from build123d import *

# Parameters (mm, degrees)
F0_W     = 3
F0_H     = 0.7113954189
F0_H_2   = 11.7951147258
F1_DEPTH = 2
F2_R     = 2
F3_W     = 4
F3_H     = 7.7592988014
F3_R     = 0.75
F4_DEPTH = 3
F5_R     = 1.99999


# Not quite as in the source:
# - a fillet or chamfer is up to 0.001 mm smaller than in the source, because OpenCascade refuses the exact size


with BuildPart() as f1:
    # F0 (on Top) → F1 (new body)
    with BuildSketch(Plane.XY):
        with BuildLine():
            ThreePointArc((-21.4, 5.9), (-20.3393398282, 6.3393398282), (-19.9, 7.4))
            Line((-19.9, 7.4), (-20.8, 7.4))
            ThreePointArc((-20.8, 7.4), (-20.9757359313, 6.9757359313), (-21.4, 6.8))
            Line((-21.4, 6.8), (-21.4, 5.9))
        make_face()
        with BuildLine():
            Line((-20.8, 7.4), (-19.9, 7.4))
            ThreePointArc((-19.9, 7.4), (-22.4606601718, 8.4606601718), (-21.4, 5.9))
            Line((-21.4, 5.9), (-21.4, 6.8))
            ThreePointArc((-21.4, 6.8), (-21.8242640687, 7.8242640687), (-20.8, 7.4))
        make_face()
        with BuildLine():
            Line((19.9, 7.4), (-19.9, 7.4))
            ThreePointArc((-19.9, 7.4), (-20.3393398282, 6.3393398282), (-21.4, 5.9))
            Line((-21.4, 5.9), (-21.4, -5.9))
            ThreePointArc((-21.4, -5.9), (-20.3393398282, -6.3393398282), (-19.9, -7.4))
            Line((-19.9, -7.4), (19.9, -7.4))
            ThreePointArc((19.9, -7.4), (20.0395252165, -6.7682497618), (20.4321444846, -6.2540263086))
            Line((20.4321444846, -6.2540263086), (20.4321444846, 6.2540263086))
            ThreePointArc((20.4321444846, 6.2540263086), (20.0395252165, 6.7682497618), (19.9, 7.4))
        make_face()
        Polygon((-1.5, 5.8975573629), (-1.5, 6.6089527819), (1.5, 6.6089527819), (1.5, 5.8975573629), (20.1555918902, 5.8975573629), (20.1555918902, -5.8975573629), (1.5, -5.8975573629), (1.5, -6.6089527819), (-1.5, -6.6089527819), (-1.5, -5.8975573629), (-20.1555918902, -5.8975573629), (-20.1555918902, 5.8975573629), align=None, mode=Mode.SUBTRACT)
        with BuildLine():
            ThreePointArc((22.9, 7.4), (21.4, 8.9), (19.9, 7.4))
            Line((19.9, 7.4), (20.8, 7.4))
            ThreePointArc((20.8, 7.4), (21.4, 8), (22, 7.4))
            ThreePointArc((22, 7.4), (21.8242640687, 6.9757359313), (21.4, 6.8))
            Line((21.4, 6.8), (21.4, 5.9))
            ThreePointArc((21.4, 5.9), (22.4606601718, 6.3393398282), (22.9, 7.4))
        make_face()
        with BuildLine():
            Line((20.8, 7.4), (19.9, 7.4))
            ThreePointArc((19.9, 7.4), (20.0395252165, 6.7682497618), (20.4321444846, 6.2540263086))
            ThreePointArc((20.4321444846, 6.2540263086), (20.8847139324, 5.9912841775), (21.4, 5.9))
            Line((21.4, 5.9), (21.4, 6.8))
            ThreePointArc((21.4, 6.8), (20.9757359313, 6.9757359313), (20.8, 7.4))
        make_face()
        with BuildLine():
            ThreePointArc((21.4, 5.9), (20.8847139324, 5.9912841775), (20.4321444846, 6.2540263086))
            Line((20.4321444846, 6.2540263086), (20.4321444846, -6.2540263086))
            ThreePointArc((20.4321444846, -6.2540263086), (20.8847139324, -5.9912841775), (21.4, -5.9))
            Line((21.4, -5.9), (21.4, 5.9))
        make_face()
        with BuildLine():
            ThreePointArc((-19.9, -7.4), (-20.3393398282, -6.3393398282), (-21.4, -5.9))
            Line((-21.4, -5.9), (-21.4, -6.8))
            ThreePointArc((-21.4, -6.8), (-20.9757359313, -6.9757359313), (-20.8, -7.4))
            Line((-20.8, -7.4), (-19.9, -7.4))
        make_face()
        with BuildLine():
            Line((-21.4, -6.8), (-21.4, -5.9))
            ThreePointArc((-21.4, -5.9), (-22.4606601718, -8.4606601718), (-19.9, -7.4))
            Line((-19.9, -7.4), (-20.8, -7.4))
            ThreePointArc((-20.8, -7.4), (-21.8242640687, -7.8242640687), (-21.4, -6.8))
        make_face()
        with BuildLine():
            ThreePointArc((21.4, -5.9), (20.8847139324, -5.9912841775), (20.4321444846, -6.2540263086))
            ThreePointArc((20.4321444846, -6.2540263086), (20.0395252165, -6.7682497618), (19.9, -7.4))
            Line((19.9, -7.4), (20.8, -7.4))
            ThreePointArc((20.8, -7.4), (20.9757359313, -6.9757359313), (21.4, -6.8))
            Line((21.4, -6.8), (21.4, -5.9))
        make_face()
        with BuildLine():
            ThreePointArc((22.9, -7.4), (22.4606601718, -6.3393398282), (21.4, -5.9))
            Line((21.4, -5.9), (21.4, -6.8))
            ThreePointArc((21.4, -6.8), (21.8242640687, -6.9757359313), (22, -7.4))
            ThreePointArc((22, -7.4), (21.4, -8), (20.8, -7.4))
            Line((20.8, -7.4), (19.9, -7.4))
            ThreePointArc((19.9, -7.4), (21.4, -8.9), (22.9, -7.4))
        make_face()
        with Locations((0, 6.2532550724)):
            Rectangle(F0_W, F0_H)
        with Locations((0, -6.2532550724)):
            Rectangle(F0_W, F0_H)
        Rectangle(F0_W, F0_H_2)
    extrude(amount=F1_DEPTH)

    # F2
    f2_edges = [f1.edges().sort_by_distance(p)[0] for p in [
        (-19.9, 7.4, 1),
        (-19.9, -7.4, 1),
        (-1.5, -5.897557, 1),
        (-20.155592, -5.897557, 1),
        (-20.155592, 5.897557, 1),
        (20.155592, 5.897557, 1),
        (20.155592, -5.897557, 1),
        (1.5, 5.897557, 1),
        (-1.5, 5.897557, 1),
        (1.5, -5.897557, 1),
        (-21.4, 5.9, 1),
        (-21.4, -5.9, 1),
        (19.9, -7.4, 1),
        (21.4, -5.9, 1),
        (21.4, 5.9, 1),
        (19.9, 7.4, 1),
    ]]
    fillet(f2_edges, radius=F2_R)

    # F3 (on face) → F4 (join, through all)
    with BuildSketch(Plane.YZ.offset(1.5)):
        with Locations((0, -1.8796494007)):
            Rectangle(F3_W, F3_H)
        with Locations((0, -3.7315103691)):
            Circle(F3_R, mode=Mode.SUBTRACT)
    extrude(amount=-F4_DEPTH)

    # F5 (radius 2 in the source; OpenCascade refuses exactly that, so slightly less here)
    f5_edges = [f1.edges().sort_by_distance(p)[0] for p in [
        (0, 2, -5.759299),
        (0, -2, -5.759299),
    ]]
    fillet(f5_edges, radius=F5_R)


solid = f1.part
Input: part model. Units: mm. Frame: model coordinates. A direction names the side the tool comes from. Coordinates: 2 decimals unless noted, no trailing zeros. Loops run counter-clockwise (first coordinate to the right, second up) from the corner with the lowest first, then second, coordinate; pieces in that order, holes last. Notation, with made-up numbers: (8.5, -39.75) - (31.5, -39.75) arc R18 cw to (31.5, -17.75) - close; hole circle Ø9 at (59.5, 44). An arc over 180 degrees is marked (long way). Answer in a Markdown table with one row per item. Add a question column.
Item 1: Access query for faces 1 (the cylindrical face through (21.6, 5.4, 1)), 2 (the cylindrical face through (2.101, 5.327, 1.014)), 3 (the flat face through (0, -7.4, 1)). Directions: +Z, -Z, +X, -X, +Y, -Y. A direction counts if a zero-diameter tool reaches every point of the face in a straight line with its end or side. Return the directions, or none.
Item 2: Mould query, pull axis X, two halves, no side actions, for faces 4 (the flat face through (0, 7.4, 1)), 5 (the flat face through (21.4, 0, 1)), 6 (the cylindrical face through (0.02, -0.55, -3.22)). Classes: released by +X, released by -X, zero draft, split by the parting line, or undercut.
Item 3: Section query C-C on x = 2.5. Return the cut outline in (y, z).
Item 4: Section query B-B on x = -16.5. Return the cut outline in (y, z).
Item 5: Contact query for flat-ended pins moving along their axis: P1, Ø0.9, axis at x = 0, z = -2.5, coming from the -Y side; P2, Ø1.4, axis at x = -21.4, y = 7.4, coming from the -Z side; P3, Ø1, axis at x = -4.5, z = 1, coming from the -Y side. Output: stop coordinate, or through.
Item 6: Section query A-A on y = 3. Return the cut outline in (x, z).
Item 7: Section query D-D on z = 1.5. State how many separate pieces and enclosed holes the cut face has, then the cut area to 3 significant figures.
Item 8: Line query: line 1 along X through (y, z) = (1.5, 1.25); line 2 along Y through (x, z) = (9, 1.5); line 3 along X through (y, z) = (-1.5, -5). Output: solid intervals per line, ascending. Write a range as [from, to].
Recorded:
| question | item | result |
|---|---|---|
| 1 | face 1 | +Z, -Z, +X |
| 1 | face 2 | +Z, -Z |
| 1 | face 3 | +Z, -Z, -Y |
| 2 | face 4 | undercut |
| 2 | face 5 | released by +X |
| 2 | face 6 | zero draft |
| 3 | outline | (-7.4, 0) - (-5.63, 0) - (-5.63, 2) - (-7.4, 2) - close; (5.63, 0) - (7.4, 0) - (7.4, 2) - (5.63, 2) - close |
| 4 | outline | (-7.4, 0) - (-5.9, 0) - (-5.9, 2) - (-7.4, 2) - close; (5.9, 0) - (7.4, 0) - (7.4, 2) - (5.9, 2) - close |
| 5 | P1 | y = -2 |
| 5 | P2 | z = 0 |
| 5 | P3 | y = -7.4 |
| 6 | outline | (-21.4, 0) - (-20.16, 0) - (-20.16, 2) - (-21.4, 2) - close; (-1.5, 0) - (1.5, 0) - (1.5, 2) - (-1.5, 2) - close; (20.16, 0) - (21.4, 0) - (21.4, 2) - (20.16, 2) - close |
| 7 | separate pieces | 1 |
| 7 | enclosed holes | 6 |
| 7 | area | 219 mm^2 |
| 8 | line 1 | [-21.4, -20.16], [-1.5, 1.5], [20.16, 21.4] |
| 8 | line 2 | [-7.4, -5.9], [5.9, 7.4] |
| 8 | line 3 | [-1.5, 1.5] |
